Here's how the part is built. I have some questions about the finished solid (model axes, mm). Face numbers are marked on the shaded views. Give positions to 0.01 mm unless a question says otherwise; leave off trailing zeros. Write each loop counter-clockwise with the first axis right and the second up, starting at its lowest first coordinate (ties: lowest second). Pieces come first, ordered by that corner, then holes. Notation, with made-up numbers: (73, -19.75) - (77, -19.75) arc R24 ccw to (77, -3.75) - close; hole circle Ø5 at (21.5, 69). An arc over 180 degrees is marked (long way). Write each question's results on one line, items separated by ' | '. Start each with the question number.
Item 1: Please list where these lines run through material, in increasing order: line 1 along X through (y, z) = (0, 7); line 2 along Y through (x, z) = (-19.5, 2.5); line 3 along Y through (x, z) = (-8, 7.75).
Item 2: Will these pins go through, and if not, where does the flat tip stop? P1, Ø2.5, axis at y = 32, z = 1.5, coming from the +X side; P2, Ø20.5, axis at x = 0, y = 0, coming from the +Z side; P3, Ø1.1, axis at y = -31.5, z = 0.5, coming from the -X side; P4, Ø1.7, axis at y = -29.5, z = 1, coming from the +X side.
Item 3: We'd pull the mould along Y, two halves only. Please class the marked faces 1 and 2: +Y half, -Y half, draft (parallel to the pull), parting line (faces both ways), or undercut.
Item 4: Suppose I cut it at A-A on z = 3. List the corners of the cut face in (x, y) for me.
Item 5: Suppose I cut it at B-B on x = 31. Count the separate pieces of the cut face and the enclosed holes in it, then the cut area to 3 significant figures.
```python
from build123d import *

# Parameters (mm, degrees)
SKETCH001_R     = 38.06
PAD_DEPTH       = 4
CHAMFER_SIZE    = 1.9
CHAMFER001_SIZE = 1.9
CHAMFER002_SIZE = 2


with BuildPart() as part:
    # Sketch → Revolution (revolve)
    with BuildSketch(Plane.XZ):
        Polygon((-17, 0), (-17, 9), (-17.8, 9), (-17.8, 7), (-28, 0.5), (-28, 0), align=None)
    revolve(axis=Axis((0, 0, 0), (0, 0, 1)))

    # Sketch001 → Pad (new body)
    with BuildSketch(Plane.XY):
        Circle(SKETCH001_R)
        with BuildLine():
            ThreePointArc((-2, 36.004494), (-25.498271, 25.498271), (-36.004494, 2))
            Line((-36.004494, 2), (-19.1, 2))
            Line((-19.1, 2), (-19.1, -2))
            Line((-19.1, -2), (-36.004494, -2))
            ThreePointArc((-36.004494, -2), (-25.498271, -25.498271), (-2, -36.004494))
            Line((-2, -36.004494), (-2, -19.1))
            Line((-2, -19.1), (2, -19.1))
            Line((2, -19.1), (2, -36.004494))
            ThreePointArc((2, -36.004494), (25.498271, -25.498271), (36.004494, -2))
            Line((19.1, -2), (36.004494, -2))
            Line((19.1, 2), (19.1, -2))
            Line((36.004494, 2), (19.1, 2))
            ThreePointArc((36.004494, 2), (25.498271, 25.498271), (2, 36.004494))
            Line((2, 36.004494), (2, 19.1))
            Line((2, 19.1), (-2, 19.1))
            Line((-2, 19.1), (-2, 36.004494))
        make_face(mode=Mode.SUBTRACT)
    extrude(amount=PAD_DEPTH)

    # Chamfer
    chamfer_edges = [part.edges().sort_by_distance(p)[0] for p in [
        (-25.498271, -25.498271, 4),
        (-25.498271, 25.498271, 4),
        (25.498271, 25.498271, 4),
        (25.498271, -25.498271, 4),
    ]]
    chamfer(chamfer_edges, length=CHAMFER_SIZE)

    # Chamfer001
    chamfer001_edges = [part.edges().sort_by_distance(p)[0] for p in [
        (-36.955885, -2, 4),
        (-29.211576, -2, 4),
        (-36.955885, 2, 4),
        (-29.211576, 2, 4),
        (-2, -29.211576, 4),
        (-2, -36.955885, 4),
        (2, -36.955885, 4),
        (2, -29.211576, 4),
        (29.211576, -2, 4),
        (36.955885, -2, 4),
        (36.955885, 2, 4),
        (29.211576, 2, 4),
        (2, 29.211576, 4),
        (2, 36.955885, 4),
        (-2, 36.955885, 4),
        (-2, 29.211576, 4),
    ]]
    chamfer(chamfer001_edges, length=CHAMFER001_SIZE)

    # Chamfer002
    chamfer002_edges = [part.edges().sort_by_distance(p)[0] for p in [
        (17, 0, 0),
    ]]
    chamfer(chamfer002_edges, length=CHAMFER002_SIZE)


solid = part.part
```
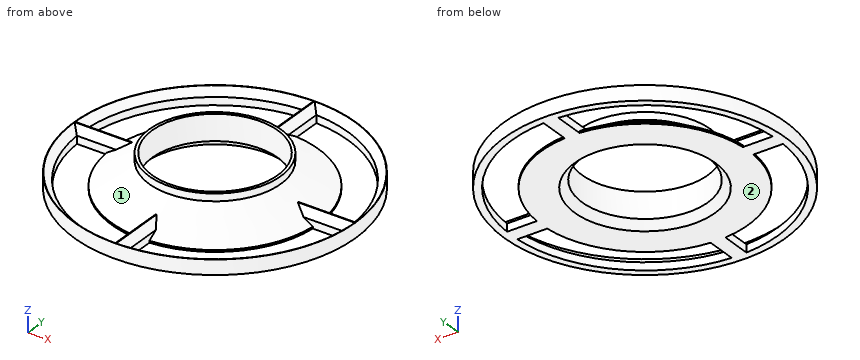
Checked values:
1) line 1: x = -17.8 to -17, 17 to 17.8 | line 2: y = -32.69 to -30.81, -15.42 to 15.42, 30.81 to 32.69 | line 3: y = -15.9 to -15, 15 to 15.9
2) P1: stops at x = 22.43 | P2: passes through | P3: stops at x = -22.15 | P4: stops at x = 25.05
3) face 1: undercut | face 2: draft
4) outline: circle Ø76.12 at (0, 0); hole (-36.94, -1.1) arc R36.96 ccw to (-1.1, -36.94) - (-1.1, -24.05) arc R24.08 cw to (-24.05, -1.1) - close; hole (-36.94, 1.1) - (-24.05, 1.1) arc R24.08 cw to (-1.1, 24.05) - (-1.1, 36.94) arc R36.96 ccw to start; hole circle Ø34 at (0, 0); hole (1.1, -36.94) arc R36.96 ccw to (36.94, -1.1) - (24.05, -1.1) arc R24.08 cw to (1.1, -24.05) - close; hole (1.1, 24.05) arc R24.08 cw to (24.05, 1.1) - (36.94, 1.1) arc R36.96 ccw to (1.1, 36.94) - close
5) separate pieces: 3 | enclosed holes: 0 | area: 34.9 mm^2
